Check sheet for the modelled part. Datum: model origin and axes. Units: mm. Give positions to 0.01 mm unless a question says otherwise; leave off trailing zeros. Loops run counter-clockwise (first coordinate to the right, second up) from the corner with the lowest first, then second, coordinate; pieces in that order, holes last. Notation, with made-up numbers: (89.5, 70) - (125.5, 70) arc R30 cw to (125.5, 106) - close; hole circle Ø3 at (-17.75, 22.5). An arc over 180 degrees is marked (long way). Answer in a Markdown table with one row per item. Add a question column.
(1) Sectioned sample at C-C on z = 0. Enter the section's corners in (x, y).
(2) Sectioned sample at D-D on y = 24. Enter the section's corners in (x, z), then the cut area to 3 significant figures.
(3) Go/stop test with flat-tipped pins: P1, Ø3, axis at x = 4, z = 121, coming from the -Y side; P2, Ø8.5, axis at y = 13.18, z = 165, coming from the -X side. Record where each tip stops, or that it passes through.
(4) Sectioned sample at B-B on x = 3.75. Enter the section's corners in (y, z), then the cut area to 3 significant figures.
(5) Thickness scan on L1, parallel to Y at x = 2, z = 145; L2, parallel to Z at x = 1.5, y = 9.5; L3, parallel to Y at x = 2.75, z = 165. Record the ranges inside material, lowest first.
(6) Sectioned sample at A-A on z = 165. Enter the section's corners in (x, y), then the cut area to 3 significant figures.
from build123d import *

# Parameters (mm, degrees)
SKETCH1_R           = 3.25
SKETCH1_R_2         = 2.75
BOSS_EXTRUDE1_DEPTH = 6.35


with BuildPart() as part:
    # Sketch1 → Boss-Extrude1 (new body)
    with BuildSketch(Plane(origin=(0, 0, 0), x_dir=(0, 0, -1), z_dir=(1, 0, 0))):
        with BuildLine():
            Line((-175.353584658, 32), (50.071343536, 32))
            Line((50.071343536, 32), (24.152715011, 0))
            Line((24.152715011, 0), (22, 0))
            ThreePointArc((22, 0), (0.91041892, 21.981154141), (-21.924648854, 1.819278055))
            Line((-21.924648854, 1.819278055), (-175.353584658, 1.819278055))
            Line((-175.353584658, 1.819278055), (-175.353584658, 32))
        make_face()
        with Locations((-165, 13.1796749)):
            Circle(SKETCH1_R, mode=Mode.SUBTRACT)
        with Locations((-145, 9.287146811)):
            Circle(SKETCH1_R_2, mode=Mode.SUBTRACT)
    extrude(amount=BOSS_EXTRUDE1_DEPTH)


solid = part.part
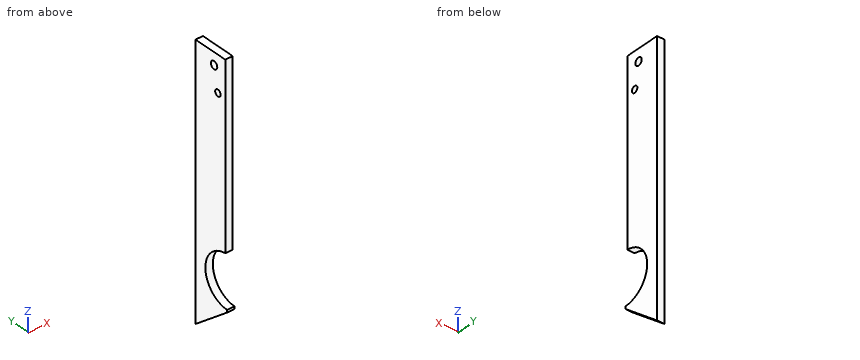
Reply:
| question | item | result |
|---|---|---|
| 1 | outline | (0, 22) - (6.35, 22) - (6.35, 32) - (0, 32) - close |
| 2 | outline | (0, -43.59) - (6.35, -43.59) - (6.35, 175.35) - (0, 175.35) - close |
| 2 | area | 1,390 mm^2 |
| 3 | P1 | y = 1.82 |
| 3 | P2 | x = 0 |
| 4 | outline | (0, -24.15) - (32, -50.07) - (32, 175.35) - (1.82, 175.35) - (1.82, 21.92) arc R22 cw to (0, -22) - close; hole circle Ø5.5 at (9.29, 145); hole circle Ø6.5 at (13.18, 165) |
| 4 | area | 5,700 mm^2 |
| 5 | L1 | 1.82 to 6.54, 12.04 to 32 |
| 5 | L2 | -31.85 to -19.84, 19.84 to 142.26, 147.74 to 175.35 |
| 5 | L3 | 1.82 to 9.93, 16.43 to 32 |
| 6 | outline | (0, 1.82) - (6.35, 1.82) - (6.35, 9.93) - (0, 9.93) - close; (0, 16.43) - (6.35, 16.43) - (6.35, 32) - (0, 32) - close |
| 6 | area | 150 mm^2 |
